```python
from build123d import *

# Parameters (mm, degrees)
SKETCH2_R                = 1.905
BOSS_EXTRUDE1_DEPTH      = 5.08
BOSS_EXTRUDE2_DEPTH      = 55
BOSS_EXTRUDE2_DEPTH_BACK = 5.08
SKETCH6_W                = 60.08
SKETCH6_H                = 8.434755733
BOSS_EXTRUDE3_DEPTH      = 2.794
BOSS_EXTRUDE4_DEPTH      = 8.434756
CHAMFER1_SIZE            = 2.54


with BuildPart() as part:
    # Sketch2 → Boss-Extrude1 (new body)
    with BuildSketch(Plane(origin=(0, 0, 0), x_dir=(0, 0, -1), z_dir=(1, 0, 0))):
        with BuildLine():
            ThreePointArc((6.35, 0), (0, -6.35), (-6.35, 0))
            add(Edge.make_bspline(
                [(-16.765082275, 10.732202813), (-10.995197474, 10.605430611), (-7.093707097, 6.823689801), (-6.35, 0)],
                knots=[0.082134521, 0.082134521, 0.082134521, 0.082134521, 1, 1, 1, 1], degree=3))
            ThreePointArc((-16.765082275, 10.732202813), (-18.143717665, 10.361153764), (-19.104415619, 9.30504185))
            ThreePointArc((-19.104415619, 9.30504185), (-20.706657527, 4.774603025), (-21.25, 0))
            ThreePointArc((-21.25, 0), (0, -21.25), (21.25, 0))
            ThreePointArc((21.25, 0), (20.706657527, 4.774603025), (19.104415619, 9.30504185))
            ThreePointArc((19.104415619, 9.30504185), (18.143717665, 10.361153764), (16.765082275, 10.732202813))
            add(Edge.make_bspline(
                [(16.765082275, 10.732202813), (10.995197474, 10.605430611), (7.093707097, 6.823689801), (6.35, 0)],
                knots=[0.082134521, 0.082134521, 0.082134521, 0.082134521, 1, 1, 1, 1], degree=3))
        make_face()
        with Locations((-15, 0)):
            Circle(SKETCH2_R, mode=Mode.SUBTRACT)
        with Locations((15, 0)):
            Circle(SKETCH2_R, mode=Mode.SUBTRACT)
    extrude(amount=BOSS_EXTRUDE1_DEPTH)

    # Sketch3 → Boss-Extrude2 (add, two sides)
    with BuildSketch(Plane.ZY) as boss_extrude2_sk:
        with BuildLine():
            ThreePointArc((16.903112003, -12.878171633), (1.771236823, -21.176052987), (-14.528859308, -15.507248215))
            Line((-14.528859308, -15.507248215), (-16.497947063, -17.608936444))
            ThreePointArc((-16.497947063, -17.608936444), (0.280682132, -24.128367486), (16.903112003, -17.220386309))
            Line((16.903112003, -17.220386309), (16.903112003, -12.878171633))
        make_face()
        with BuildLine():
            ThreePointArc((16.903112003, -8.785630576), (3.210032128, -18.777598189), (-13.02469505, -13.90179193))
            Line((-13.02469505, -13.90179193), (-14.528859308, -15.507248215))
            ThreePointArc((-14.528859308, -15.507248215), (1.771236823, -21.176052987), (16.903112003, -12.878171633))
            Line((16.903112003, -12.878171633), (16.903112003, -8.785630576))
        make_face()
    extrude(amount=BOSS_EXTRUDE2_DEPTH)
    extrude(boss_extrude2_sk.sketch, amount=-BOSS_EXTRUDE2_DEPTH_BACK)

    # Sketch6 → Boss-Extrude3 (add)
    with BuildSketch(Plane.XY.offset(16.903112003)):
        with Locations((-24.96, -13.003008443)):
            Rectangle(SKETCH6_W, SKETCH6_H)
    extrude(amount=BOSS_EXTRUDE3_DEPTH)

    # Sketch7 → Boss-Extrude4 (add)
    with BuildSketch(Plane(origin=(0, -8.785630576, 0), x_dir=(1, 0, 0), z_dir=(0, 1, 0))):
        Polygon((-53.728777932, -19.697112003), (-53.728777932, -29.222112003), (-4.829590455, -29.222112003), (5.08, -19.697112003), align=None)
        Polygon((-50.534168456, -22.645679195), (-48.67304704, -20.078112003), (-6.76304704, -20.078112003), (-6.76304704, -25.412112003), (-48.67304704, -25.412112003), (-50.534168456, -22.84454481), align=None, mode=Mode.SUBTRACT)
    extrude(amount=-BOSS_EXTRUDE4_DEPTH)

    # Chamfer1
    chamfer1_edges = [part.edges().sort_by_distance(p)[0] for p in [
        (-53.728777932, -13.003008576, 29.222112003),
    ]]
    chamfer(chamfer1_edges, length=CHAMFER1_SIZE)


solid = part.part
```
Could you check a few things on this model? Use its own coordinates, in mm. A direction names the side the tool comes from. Round coordinates to 2 decimals unless told otherwise and drop trailing zeros. Write each loop counter-clockwise with the first axis right and the second up, starting at its lowest first coordinate (ties: lowest second). Pieces come first, ordered by that corner, then holes. Notation, with made-up numbers: M 60,50 L 98,50 A11 ccw 98,71 Z; hole C 69,82 d1. An arc over 180 degrees is marked long. Answer in a Markdown table with one row per item. Add a question column.
Q1. Imagine slicing it at B-B (y = -13). Please give me the cut outline in (x, z), then the cut area to 3 significant figures.
Q2. Will these pins go through, and if not, where does the flat tip stop? pin 1 Ø5 at (x, z) = (-48, -8) entering from -Y; pin 2 Ø1 at (y, z) = (2.5, -16) entering from -X; pin 3 Ø4 at (x, z) = (-47, 7) entering from +Y.
Q3. Imagine slicing it at C-C (z = 2.5). Please give me the cut outline in (x, y), then the cut area to 3 significant figures.
Q4. If we mould it in two halves opening along Y, with no side actions, what happens to faces 5 (the flat face through (-28, -13, 20.078)), 6 (the cylindrical face through (-25.38, -24.13, 0.02)), 7 (the cylindrical face through (2.5, -0.73, -16.76))? For each: +Y half, -Y half, draft (parallel to the pull), parting line (faces both ways), or undercut.
Q5. If I drill on line 1 (Y direction, x = 1.15, z = -15) (3 decimals); line 2 (X direction, y = 1.5, z = 20); line 3 (Z direction, x = -17.5, y = -13.5), over which ranges is the centre line in solid material (lowest first)? Write a range as from..to.
Q6. On a 3-axis mill with a long thin cutter (end or side, diameter ignored), from which of +Z, -Z, +X, -X, +Y, -Y can I reach the whole of each face in a straight line? I mean faces 1 (the flat face through (-27, -13, 25.412)), 2 (the cylindrical face through (-27.115, -18.735, 3.452)), 3 (the cylindrical face through (2.5, -6.35, -0.14)), 4 (the flat face through (-53.729, -13, 23)). Say none if no direction works.
Q7. Imagine slicing it at A-A (x = -11.5). Please give me the cut outline in (y, z).
Q8. Imagine slicing it at D-D (x = -1). Please give me the cut outline in (y, z), then the cut area to 3 significant figures.
Values:
| question | item | result |
|---|---|---|
| 1 | outline | M -55,13.92 L 0,13.92 L 0,-16.81 L 5.08,-16.81 L 5.08,19.7 L -4.83,29.22 L -51.19,29.22 L -53.73,26.68 L -53.73,19.7 L -55,19.7 Z; hole M -50.53,22.65 L -48.67,20.08 L -6.76,20.08 L -6.76,25.41 L -48.67,25.41 L -50.53,22.84 Z |
| 1 | area | 784 mm^2 |
| 2 | pin 1 | y = -23.49 |
| 2 | pin 2 | x = 0 |
| 2 | pin 3 | y = -16.79 |
| 3 | outline | M -55,-24 L 5.08,-24 L 5.08,-5.84 L 0,-5.84 L 0,-18.89 L -55,-18.89 Z |
| 3 | area | 374 mm^2 |
| 4 | face 5 | draft |
| 4 | face 6 | -Y half |
| 4 | face 7 | undercut |
| 5 | line 1 | -18.901..-16.01, -15.052..-1.905, 1.905..10.57 |
| 5 | line 2 | 0..5.08 |
| 5 | line 3 | 13.44..20.08, 25.41..29.22 |
| 6 | face 1 | +Y, -Y |
| 6 | face 2 | -X, +Y |
| 6 | face 3 | +X, -X, +Y |
| 6 | face 4 | +Z, -X, +Y, -Y |
| 7 | outline | M -17.61,-16.5 L -13.9,-13.02 A19.05 cw -8.79,16.9 L -8.79,20.08 L -17.22,20.08 L -17.22,16.9 A24.13 ccw Z; M -17.22,25.41 L -8.79,25.41 L -8.79,29.22 L -17.22,29.22 Z |
| 8 | outline | M -17.61,-16.5 L -13.9,-13.02 A19.05 cw -8.79,16.9 L -8.79,25.54 L -17.22,25.54 L -17.22,16.9 A24.13 ccw Z |
| 8 | area | 255 mm^2 |
